from build123d import *

# Parameters (mm, degrees)
F0_R     = 3.175
F0_R_2   = 72.39
F1_DEPTH = 6.35
F2_DEPTH = 50.8
F3_DEPTH = 57.15
F4_DEPTH = 57.15


with BuildPart() as f1:
    # F0 (on Top) → F1 (new body)
    with BuildSketch(Plane.XY):
        with BuildLine():
            Line((-63.0026039546, 52.3520689175), (-63.0026039546, 118.4635039546))
            ThreePointArc((-63.0026039546, 118.4635039546), (-68.1927298466, 117.4311237264), (-71.1327, 121.8311))
            Line((-71.1327, 121.8311), (-71.1327, 40.6227302838))
            ThreePointArc((-71.1327, 40.6227302838), (-81.915, 0), (-71.1327, -40.6227302838))
            Line((-71.1327, -40.6227302838), (-71.1327, -121.8311))
            ThreePointArc((-71.1327, -121.8311), (-68.1927298466, -117.4311237264), (-63.0026039546, -118.4635039546))
            Line((-63.0026039546, -118.4635039546), (-63.0026039546, -52.3520689175))
            ThreePointArc((-63.0026039546, -52.3520689175), (0, -81.915), (63.0026039546, -52.3520689175))
            Line((63.0026039546, -52.3520689175), (63.0026039546, -118.4635039546))
            ThreePointArc((63.0026039546, -118.4635039546), (68.1927298466, -117.4311237264), (71.1327, -121.8311))
            Line((71.1327, -121.8311), (71.1327, -40.6227302838))
            ThreePointArc((71.1327, -40.6227302838), (81.915, 0), (71.1327, 40.6227302838))
            Line((71.1327, 40.6227302838), (71.1327, 121.8311))
            ThreePointArc((71.1327, 121.8311), (68.1927298466, 117.4311237264), (63.0026039546, 118.4635039546))
            Line((63.0026039546, 118.4635039546), (63.0026039546, 52.3520689175))
            ThreePointArc((63.0026039546, 52.3520689175), (0, 81.915), (-63.0026039546, 52.3520689175))
        make_face()
        with Locations((0, -75.7809)):
            Circle(F0_R, mode=Mode.SUBTRACT)
        with Locations((-75.7809, 0)):
            Circle(F0_R, mode=Mode.SUBTRACT)
        Circle(F0_R_2, mode=Mode.SUBTRACT)
        with Locations((75.7809, 0)):
            Circle(F0_R, mode=Mode.SUBTRACT)
        with Locations((0, 75.7809)):
            Circle(F0_R, mode=Mode.SUBTRACT)
    extrude(amount=F1_DEPTH)



with BuildPart() as f1b:
    # F0 (on Top) → F1, piece 2 (new body)
    with BuildSketch(Plane.XY):
        with BuildLine():
            ThreePointArc((-61.6077, 121.8311), (-61.9702237264, 120.0085701534), (-63.0026039546, 118.4635039546))
            Line((-63.0026039546, 118.4635039546), (63.0026039546, 118.4635039546))
            ThreePointArc((63.0026039546, 118.4635039546), (61.9702237264, 123.6536298466), (66.3702, 126.5936))
            Line((66.3702, 126.5936), (-66.3702, 126.5936))
            ThreePointArc((-66.3702, 126.5936), (-63.0026039546, 125.1986960454), (-61.6077, 121.8311))
        make_face()
    extrude(amount=F1_DEPTH)


with BuildPart() as f1c:
    # F0 (on Top) → F1, piece 3 (new body)
    with BuildSketch(Plane.XY):
        with BuildLine():
            Line((63.0026039546, -118.4635039546), (-63.0026039546, -118.4635039546))
            ThreePointArc((-63.0026039546, -118.4635039546), (-61.9702237264, -120.0085701534), (-61.6077, -121.8311))
            ThreePointArc((-61.6077, -121.8311), (-63.0026039546, -125.1986960454), (-66.3702, -126.5936))
            Line((-66.3702, -126.5936), (66.3702, -126.5936))
            ThreePointArc((66.3702, -126.5936), (61.9702237264, -123.6536298466), (63.0026039546, -118.4635039546))
        make_face()
    extrude(amount=F1_DEPTH)


with BuildPart() as f1d:
    # F0 (on Top) → F1, piece 4 (new body)
    with BuildSketch(Plane.XY):
        with BuildLine():
            ThreePointArc((-66.3702, -126.5936), (-69.7377960454, -125.1986960454), (-71.1327, -121.8311))
            Line((-71.1327, -121.8311), (-71.1327, -126.5936))
            Line((-71.1327, -126.5936), (-66.3702, -126.5936))
        make_face()
    extrude(amount=F1_DEPTH)


with BuildPart() as f1e:
    # F0 (on Top) → F1, piece 5 (new body)
    with BuildSketch(Plane.XY):
        with BuildLine():
            Line((71.1327, -126.5936), (71.1327, -121.8311))
            ThreePointArc((71.1327, -121.8311), (69.7377960454, -125.1986960454), (66.3702, -126.5936))
            Line((66.3702, -126.5936), (71.1327, -126.5936))
        make_face()
    extrude(amount=F1_DEPTH)


with BuildPart() as f1f:
    # F0 (on Top) → F1, piece 6 (new body)
    with BuildSketch(Plane.XY):
        with BuildLine():
            Line((-71.1327, 126.5936), (-71.1327, 121.8311))
            ThreePointArc((-71.1327, 121.8311), (-69.7377960454, 125.1986960454), (-66.3702, 126.5936))
            Line((-66.3702, 126.5936), (-71.1327, 126.5936))
        make_face()
    extrude(amount=F1_DEPTH)


with BuildPart() as f1g:
    # F0 (on Top) → F1, piece 7 (new body)
    with BuildSketch(Plane.XY):
        with BuildLine():
            ThreePointArc((66.3702, 126.5936), (69.7377960454, 125.1986960454), (71.1327, 121.8311))
            Line((71.1327, 121.8311), (71.1327, 126.5936))
            Line((71.1327, 126.5936), (66.3702, 126.5936))
        make_face()
    extrude(amount=F1_DEPTH)


with BuildPart() as f1_1:
    add(f1.part)

    add(f1b.part)  # F2 merges F1b

    add(f1c.part)  # F2 merges F1c

    add(f1d.part)  # F2 merges F1d

    add(f1e.part)  # F2 merges F1e

    add(f1f.part)  # F2 merges F1f

    add(f1g.part)  # F2 merges F1g
    # F0 (on Top) → F2 (join)
    with BuildSketch(Plane.XY):
        with BuildLine():
            ThreePointArc((-71.1327, 121.8311), (-68.1927298466, 117.4311237264), (-63.0026039546, 118.4635039546))
            ThreePointArc((-63.0026039546, 118.4635039546), (-61.9702237264, 120.0085701534), (-61.6077, 121.8311))
            ThreePointArc((-61.6077, 121.8311), (-63.0026039546, 125.1986960454), (-66.3702, 126.5936))
            ThreePointArc((-66.3702, 126.5936), (-69.7377960454, 125.1986960454), (-71.1327, 121.8311))
        make_face()
        with Locations((-66.3702, 121.8311)):
            Circle(F0_R, mode=Mode.SUBTRACT)
        with BuildLine():
            ThreePointArc((66.3702, 126.5936), (61.9702237264, 123.6536298466), (63.0026039546, 118.4635039546))
            ThreePointArc((63.0026039546, 118.4635039546), (68.1927298466, 117.4311237264), (71.1327, 121.8311))
            ThreePointArc((71.1327, 121.8311), (69.7377960454, 125.1986960454), (66.3702, 126.5936))
        make_face()
        with Locations((66.3702, 121.8311)):
            Circle(F0_R, mode=Mode.SUBTRACT)
        with BuildLine():
            ThreePointArc((-63.0026039546, -118.4635039546), (-68.1927298466, -117.4311237264), (-71.1327, -121.8311))
            ThreePointArc((-71.1327, -121.8311), (-69.7377960454, -125.1986960454), (-66.3702, -126.5936))
            ThreePointArc((-66.3702, -126.5936), (-63.0026039546, -125.1986960454), (-61.6077, -121.8311))
            ThreePointArc((-61.6077, -121.8311), (-61.9702237264, -120.0085701534), (-63.0026039546, -118.4635039546))
        make_face()
        with Locations((-66.3702, -121.8311)):
            Circle(F0_R, mode=Mode.SUBTRACT)
        with BuildLine():
            ThreePointArc((66.3702, -126.5936), (69.7377960454, -125.1986960454), (71.1327, -121.8311))
            ThreePointArc((71.1327, -121.8311), (68.1927298466, -117.4311237264), (63.0026039546, -118.4635039546))
            ThreePointArc((63.0026039546, -118.4635039546), (61.9702237264, -123.6536298466), (66.3702, -126.5936))
        make_face()
        with Locations((66.3702, -121.8311)):
            Circle(F0_R, mode=Mode.SUBTRACT)
    extrude(amount=F2_DEPTH)

    # F0 (on Top) → F3 (join)
    with BuildSketch(Plane.XY):
        with Locations((66.3702, -121.8311)):
            Circle(F0_R)
        with Locations((-66.3702, -121.8311)):
            Circle(F0_R)
        with Locations((66.3702, 121.8311)):
            Circle(F0_R)
        with Locations((-66.3702, 121.8311)):
            Circle(F0_R)
    extrude(amount=F3_DEPTH)

    # F0 (on Top) → F4 (join)
    with BuildSketch(Plane.XY):
        with Locations((0, 75.7809)):
            Circle(F0_R)
        with Locations((-75.7809, 0)):
            Circle(F0_R)
        with Locations((75.7809, 0)):
            Circle(F0_R)
        with Locations((0, -75.7809)):
            Circle(F0_R)
    extrude(amount=F4_DEPTH)


solid = f1_1.part
The listing builds one solid part. Answer for the finished solid, in the listing's coordinates (mm). A direction names the side the tool comes from. Give positions to 0.01 mm unless a question says otherwise; leave off trailing zeros. Loops run counter-clockwise (first coordinate to the right, second up) from the corner with the lowest first, then second, coordinate; pieces in that order, holes last. Notation, with made-up numbers: (8, -10) - (12, -10) arc R23 ccw to (12, 15) - close; hole circle Ø7 at (15, 88.5). An arc over 180 degrees is marked (long way). Use one line per item in the form item = value.
1. Section D-D on y = 0 is taken. Give the vertices of the cut face in (x, z) (3 decimals), then the cut area to 3 significant figures.
Calculated:
outline = (-81.915, 0) - (-72.39, 0) - (-72.39, 6.35) - (-72.606, 6.35) - (-72.606, 57.15) - (-78.956, 57.15) - (-78.956, 6.35) - (-81.915, 6.35) - close; (72.39, 0) - (81.915, 0) - (81.915, 6.35) - (78.956, 6.35) - (78.956, 57.15) - (72.606, 57.15) - (72.606, 6.35) - (72.39, 6.35) - close
area = 766 mm^2
2. Given pin 1 Ø7 at (y, z) = (-71.5, 3) entering from +X; pin 2 Ø10 at (y, z) = (-5.5, 26.5) entering from +X; pin 3 Ø7 at (y, z) = (-97.5, 4.5) entering from -X, each flat-ended and moving along its own axis, determine where each tip first touches the part or whether it passes through.
Calculated:
pin_1 = 71.13
pin_2 = 78.92
pin_3 = -71.13
3. Section A-A on y = -92.5 is taken. Give the vertices of the cut face in (x, z).
Calculated:
outline = (-71.13, 0) - (-63, 0) - (-63, 6.35) - (-71.13, 6.35) - close; (63, 0) - (71.13, 0) - (71.13, 6.35) - (63, 6.35) - close
4. Section B-B on x = 0 is taken. Count the separate pieces of the cut face and the enclosed holes in it, then the cut area to 3 significant figures.
Calculated:
separate_pieces = 4
enclosed_holes = 0
area = 869 mm^2
5. Find the intervals of material crossed by line 1 along Y through (x, z) = (0, 5.25) (1 decimal); line 2 along Z through (x, y) = (-63.5, -93); line 3 along X through (y, z) = (75, 53.5), in increasing order. Write a range as [from, to].
Calculated:
line_1 = [-126.6, -118.5], [-81.9, -72.4], [72.4, 81.9], [118.5, 126.6]
line_2 = [0, 6.35]
line_3 = [-3.08, 3.08]
6. The mould has two halves that part along X. Classify faces 1 (the face through (-71.133, 84, 3)), 2 (the face through (1, -118.464, 3)), 3 (the face through (-63.003, 85, 3)), 4 (the face through (-66, 122, 57.15)): pulls with the +X half, pulls with the -X half, needs draft (parallel to the pull), parting line crosses it, or undercut.
Calculated:
face_1 = pulls with the -X half
face_2 = undercut
face_3 = undercut
face_4 = needs draft
7. Which of the six approach directions +Z, -Z, +X, -X, +Y, -Y give full straight-line access (tool end or side, diameter ignored) to faces 5 (the face through (-70.2, 125.5, 6.35)), 6 (the face through (-63.003, -86, 3)), 7 (the face through (-61.828, -120.401, 28.264)), 8 (the face through (-76, 0, 57.15))?
Calculated:
face_5 = +Z, -X, +Y
face_6 = +Z, -Z
face_7 = +Z
face_8 = +Z, +X, -X, +Y, -Y
